Design review of the part built by this model. Coordinates are the model's own, in mm. A direction names the side the tool comes from. Coordinates: 2 decimals unless noted, no trailing zeros. Order: outer loops, then holes, each group sorted by start corner. A loop starts at its lowest first (then second) coordinate and runs counter-clockwise, first axis right, second up. Notation, with made-up numbers: (1, 83) -> (11, 83) arc R18 ccw to (11, 112) -> close; hole circle Ø10 at (-28.75, -1). An arc over 180 degrees is marked (long way). Write item = value, one per line.
```python
from build123d import *

# Parameters (mm, degrees)
F0_R     = 8
F0_R_2   = 6
F1_DEPTH = 53.3
F2_DEPTH = 6
F3_START = 6
F3_DEPTH = 3.7
F4_SIZE  = 8
F5_D     = 4
F5_DEPTH = 20
F5_TIP   = 1.2017212381
F6_D     = 0.4
F6_DEPTH = 70
F6_TIP   = 0.1201721238


with BuildPart() as f1:
    # F0 (on Top) → F1 (new body)
    with BuildSketch(Plane.XY):
        with Locations((-42.3969104886, 33.1056714058)):
            Circle(F0_R)
        with Locations((-42.3969104886, 33.1056714058)):
            Circle(F0_R_2, mode=Mode.SUBTRACT)
        with Locations((-42.3969104886, 33.1056714058)):
            Circle(F0_R_2)
    extrude(amount=-F1_DEPTH)

    # F0 (on Top) → F2 (join)
    with BuildSketch(Plane.XY):
        with Locations((-42.3969104886, 33.1056714058)):
            Circle(F0_R_2)
    extrude(amount=F2_DEPTH)

    # F0 (on Top) → F3 (join)
    with BuildSketch(Plane.XY.offset(F3_START)):
        with Locations((-42.3969104886, 33.1056714058)):
            Circle(F0_R)
        with Locations((-42.3969104886, 33.1056714058)):
            Circle(F0_R_2, mode=Mode.SUBTRACT)
        with Locations((-42.3969104886, 33.1056714058)):
            Circle(F0_R_2)
    extrude(amount=F3_DEPTH)

    # F4
    f4_edges = [f1.edges().sort_by_distance(p)[0] for p in [
        (-50.39691, 33.105671, -53.3),
    ]]
    chamfer(f4_edges, length=F4_SIZE)

    # F5 (one way)
    with BuildSketch(Plane(origin=(0, 0, 0), x_dir=(1, 0, 0), z_dir=(0, 0, -1))):
        with Locations((-42.3969104886, -33.1056714058)):
            Circle(F5_D / 2)
    extrude(amount=-F5_DEPTH, mode=Mode.SUBTRACT)
    with Locations(Plane(origin=(0, 0, 0), x_dir=(1, 0, 0), z_dir=(0, 0, -1))):
        with Locations((-42.3969104886, -33.1056714058)):
            with Locations((0, 0, -(F5_DEPTH + F5_TIP / 2))):  # 118° drill point
                Cone(0, F5_D / 2, F5_TIP, mode=Mode.SUBTRACT)

    # F6
    with Locations(Plane.XY):
        with Locations((-42.3969104886, 33.1056714058)):
            Hole(F6_D / 2, depth=F6_DEPTH)
            with Locations((0, 0, -(F6_DEPTH + F6_TIP / 2))):  # 118° drill point
                Cone(0, F6_D / 2, F6_TIP, mode=Mode.SUBTRACT)


solid = f1.part
```
(1) We need section A-A (z = -4.5). Write out the cut boundary in (x, y).
Report:
outline = circle Ø16 at (-42.4, 33.11); hole circle Ø0.4 at (-42.4, 33.11)
(2) The part is to be moulded in two halves that separate along X. For faces 3 (the flat face through (-44.2, 39.1, 0)), 4 (the cylindrical face through (-43.7, 27.25, 2.96)), 5 (the flat face through (-42, 33, 0)), 6 (the cylindrical face through (-42.83, 35.06, 4.78)), say which applies: released by +X, released by -X, zero draft, split by the parting line, or undercut.
Report:
face_3 = zero draft
face_4 = split by the parting line
face_5 = undercut
face_6 = undercut
(3) For faces 1 (the cylindrical face through (-34.766, 35.509, -22.333)), 2 (the flat face through (-44.2, 39.1, 6)), list the 3-axis set-ups (+Z, -Z, +X, -X, +Y, -Y) from which the entire face can be reached by the end or side of a thin tool; tool diameter is ignored.
Report:
face_1 = +Z, -Z
face_2 = none
(4) For L1, parallel to Y at x = -42.75, z = -43; L2, parallel to Z at x = -36.5, y = 37.75; L3, parallel to Z at x = -41.75, y = 33.25, list the stretches that pass through material, from the lowest coordinate up.
Report:
L1 = 25.11 to 41.1
L2 = -45.79 to 0, 6 to 9.7
L3 = -52.64 to 0
(5) Insertion check: pin 1 (6 mm diameter, centred on x = -48, z = -23, fed in from -Y); pin 2 (1.5 mm diameter, centred on y = 36, z = -22.5, fed in from +X); pin 3 (3.5 mm diameter, centred on x = -42.4, y = 33.11, fed in from -Z); pin 4 (1.5 mm diameter, centred on x = -41, y = 29, fed in from -Z). Each pin has a flat end and moves straight along its axis. Give the tip position at first contact, or say it passes through.
Report:
pin_1 = 25.54
pin_2 = -34.69
pin_3 = -53.1
pin_4 = -49.71
